```python
from build123d import *

# Parameters (mm, degrees)
SKETCH1_W             = 40
SKETCH1_H             = 40
BOSS_EXTRUDE1_DEPTH   = 48
M4X0_7_TAPPED_HOLE1_D = 3.3
SKETCH10_W            = 40
SKETCH10_H            = 20
CUT_EXTRUDE4_DEPTH    = 49
SKETCH11_W            = 11.25
SKETCH11_H            = 7.2
CUT_EXTRUDE5_REACH    = 50
SKETCH12_R            = 10
M4X0_7_TAPPED_HOLE2_D = 3.3
SKETCH15_W            = 40
SKETCH15_H            = 7.5
CUT_EXTRUDE6_DEPTH    = 36


with BuildPart() as part:
    # Sketch1 → Boss-Extrude1 (new body)
    with BuildSketch(Plane(origin=(0, 0, 0), x_dir=(1, 0, 0), z_dir=(0, 1, 0))):
        Rectangle(SKETCH1_W, SKETCH1_H)
    extrude(amount=-BOSS_EXTRUDE1_DEPTH)

    # M4x0.7 Tapped Hole1 (through all)
    with Locations(Plane(origin=(0, 0, 0), x_dir=(1, 0, 0), z_dir=(0, 1, 0))):
        with Locations((-15.5, 16), (15.5, 16), (15.5, -16), (-15.5, -16)):
            Hole(M4X0_7_TAPPED_HOLE1_D / 2)

    # Sketch10 → Cut-Extrude4 (cut, through all)
    with BuildSketch(Plane(origin=(0, 0, 0), x_dir=(1, 0, 0), z_dir=(0, 1, 0))):
        with Locations((0, -10)):
            Rectangle(SKETCH10_W, SKETCH10_H)
    extrude(amount=-CUT_EXTRUDE4_DEPTH, mode=Mode.SUBTRACT)

    # Sketch11 → Cut-Revolve2 (revolve, cut)
    with BuildSketch(Plane.XY):
        with Locations((5.625, -43.6)):
            Rectangle(SKETCH11_W, SKETCH11_H)
    revolve(axis=Axis((0, 0, 0), (0, -1, 0)), mode=Mode.SUBTRACT)

    # Sketch12 → Cut-Extrude5 (cut, up to next)
    with BuildSketch(Plane.XZ.offset(48), mode=Mode.PRIVATE) as cut_extrude5_sk1:
        Circle(SKETCH12_R)
    cut_extrude5_tool1 = extrude(cut_extrude5_sk1.sketch, amount=-CUT_EXTRUDE5_REACH, mode=Mode.PRIVATE) & part.part
    add(cut_extrude5_tool1.solids().sort_by_distance((0, -48, 0))[0], mode=Mode.SUBTRACT)

    # M4x0.7 Tapped Hole2 (through all)
    with Locations(Plane(origin=(0, 0, -20), x_dir=(-1, 0, 0), z_dir=(0, 0, -1))):
        with Locations((15, -43.628125), (-15, -43.628125), (0, -36.484375), (0, -18.2421875)):
            Hole(M4X0_7_TAPPED_HOLE2_D / 2)

    # Sketch15 → Cut-Extrude6 (cut)
    with BuildSketch(Plane.XZ.offset(48)):
        with Locations((0, -16.25)):
            Rectangle(SKETCH15_W, SKETCH15_H)
    extrude(amount=-CUT_EXTRUDE6_DEPTH, mode=Mode.SUBTRACT)


solid = part.part
```
Geometry: final body of the model. Coordinates: model frame, mm. A direction names the side the tool comes from. Round coordinates to 2 decimals unless told otherwise and drop trailing zeros. Order: outer loops, then holes, each group sorted by start corner. A loop starts at its lowest first (then second) coordinate and runs counter-clockwise, first axis right, second up. Notation, with made-up numbers: (61, 20) - (77, 20) arc R21 cw to (77, 29) - close; hole circle Ø6 at (-36, 50). An arc over 180 degrees is marked (long way). Write item = value, one per line. Start each with the question number.
Q1. Access query for faces 5 (the flat face through (0, 0, -10)), 6 (the flat face through (0, -12, -16)), 7 (the cylindrical face through (13.976, -6.084, -15.368)), 8 (the cylindrical face through (-0.2, -47.6, -10)), 9 (the flat face through (0.1, -47.2, -10.2)). Directions: +Z, -Z, +X, -X, +Y, -Y. A direction counts if a zero-diameter tool reaches every point of the face in a straight line with its end or side. Return the directions, or none.
Q2. Cut plane A-A on z = -16. Return the cut outline in (x, y).
Q3. Cut plane B-B on x = 0. Return the cut outline in (y, z), and give its area (4 significant figures).
Q4. Cut plane D-D on z = -6.5. Return the cut outline in (x, y).
Q5. Cut plane C-C on y = -7. Return the cut outline in (x, z).
Q6. Pull-direction query (X, two-part tool) for faces 1 (the cylindrical face through (15.89, -42.24, -6.16)), 2 (the cylindrical face through (-0.247, -43.55, -11.247)), 3 (the flat face through (0, -30, -12.5)), 4 (the flat face through (-20, -24, -8)); classes: +X half, -X half, draft (parallel to the pull), parting line (faces both ways), or undercut.
Q7. Pin query (flat end, axial travel): pin 1 (4 mm diameter, centred on x = 0, y = -36.48, fed in from -Z); pin 2 (1 mm diameter, centred on x = -2.5, z = -13.5, fed in from -Y); pin 3 (3 mm diameter, centred on x = 15, y = -43.63, fed in from -Z); pin 4 (3.5 mm diameter, centred on x = 1, z = -4, fed in from -Y). Return the tip coordinate at first contact, or that it passes through.
Q8. Ray query, line 1 (Y direction, x = 0, z = -8.5); line 2 (Y direction, x = -15, z = -6); line 3 (Z direction, x = 15.5, y = -5.75). Return the intervals inside material, ascending. Write a range as from..to.
Outcome:
q1.face_5 = +Z, -Z, +X, -X, +Y
q1.face_6 = -Z, +X, -X, -Y
q1.face_7 = +Y, -Y
q1.face_8 = +Z, -Y
q1.face_9 = +Z
q2.outline = (-20, -12) - (-17.15, -12) - (-17.15, 0) - (-20, 0) - close; (-13.85, -12) - (13.85, -12) - (13.85, 0) - (-13.85, 0) - close; (17.15, -12) - (20, -12) - (20, 0) - (17.15, 0) - close
q3.outline = (-48, -12.5) - (-38.13, -12.5) - (-38.13, 0) - (-40, 0) - (-40, -11.25) - (-47.2, -11.25) - (-47.2, -10) - (-48, -10) - close; (-34.83, -12.5) - (-19.89, -12.5) - (-19.89, 0) - (-34.83, 0) - close; (-16.59, -12.5) - (-12, -12.5) - (-12, -20) - (0, -20) - (0, 0) - (-16.59, 0) - close
q3.area = 518.5 mm^2
q4.outline = (-20, -48) - (-7.6, -48) - (-7.6, -47.2) - (-9.18, -47.2) - (-9.18, -40) - (9.18, -40) - (9.18, -47.2) - (7.6, -47.2) - (7.6, -48) - (20, -48) - (20, 0) - (-20, 0) - close; hole circle Ø3.3 at (-15, -43.63); hole circle Ø3.3 at (0, -36.48); hole circle Ø3.3 at (0, -18.24); hole circle Ø3.3 at (15, -43.63)
q5.outline = (-20, -20) - (20, -20) - (20, 0) - (-20, 0) - close; hole circle Ø3.3 at (-15.5, -16); hole circle Ø3.3 at (15.5, -16)
q6.face_1 = undercut
q6.face_2 = undercut
q6.face_3 = draft
q6.face_4 = -X half
q7.pin_1 = -12.5
q7.pin_2 = -12
q7.pin_3 = through
q7.pin_4 = -40
q8.line_1 = -40..-38.13, -34.83..-19.89, -16.59..0
q8.line_2 = -48..-45.28, -41.98..0
q8.line_3 = -20..-17.65, -14.35..0
